Here's how the part is built. I have some questions about the finished solid (model axes, mm). Face numbers are marked on the shaded views. A direction names the side the tool comes from. Give positions to 0.01 mm unless a question says otherwise; leave off trailing zeros. Order: outer loops, then holes, each group sorted by start corner. A loop starts at its lowest first (then second) coordinate and runs counter-clockwise, first axis right, second up. Notation, with made-up numbers: (-5.5, -28.75) -> (34.5, -28.75) arc R36 ccw to (34.5, 7.25) -> close; hole circle Ø8 at (-13.5, 85.5). An arc over 180 degrees is marked (long way). Write each question's results on one line, items separated by ' | '. Start each with the question number.
Q1. Imagine slicing it at C-C, the plane x = -4.5. Please give me the cut outline in (y, z).
Q2. I need wall thicknesses on line 1 along X through (y, z) = (-10.5, 1.05); line 2 along Y through (x, z) = (15.25, -1.1); line 3 along Y through (x, z) = (15.25, 0.6). Which ranges of each line are inside material? Lowest first, please. Write a range as [from, to].
Q3. Imagine slicing it at B-B, the plane z = -3.15. State how many separate pieces and enclosed holes the cut face has, then the cut area to 3 significant figures.
Q4. Imagine slicing it at A-A, the plane y = -7.5. Please give me the cut outline in (x, z).
Q5. Thinking about a two-plate mould opening in X: for the marked faces 1, 2 and 3, which applies, pulls with the +X half, pulls with the -X half, needs draft (parallel to the pull), parting line crosses it, or undercut?
Q6. For the marked faces 4, 5 and 6, which set-ups out of +Z, -Z, +X, -X, +Y, -Y let a thin tool reach every point of the face, with its end or its side?
Q7. I'm going to push flat-ended pins straight in: pin 1 (2 mm diameter, centred on x = 4, z = -0.5, fed in from -Y); pin 2 (2 mm diameter, centred on y = 5, z = -2.5, fed in from -X); pin 3 (3 mm diameter, centred on x = 8, y = -2.5, fed in from -Z). Where does each tip first touch, or does it pass through?
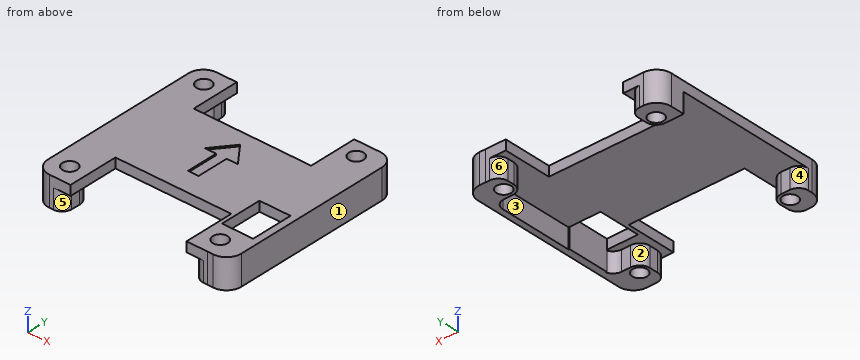
```python
from build123d import *

# Parameters (mm, degrees)
F0_R         = 1.5
F1_DEPTH     = 2
F2_DEPTH     = 4
F3_T1_DEPTH  = 9
F4_T4_DEPTH  = 9
F4_T6_DEPTH  = 4
F4_T8_DEPTH  = 9
F4_T10_DEPTH = 8.8612846748
F4_T12_DEPTH = 9
F4_T14_DEPTH = 9
F5_R         = 3
F6_R         = 3
F8_DEPTH     = 0.3


# Not quite as in the source:
# - a fillet or chamfer that OpenCascade refuses, or shapes differently, is made with other operations: its cross-section is extruded or revolved along the edge and cut away or added


with BuildPart() as f1:
    # F0 (on Top) → F1 (new body)
    with BuildSketch(Plane.XY):
        with BuildLine():
            Line((11.75, -19), (13.2, -19))
            Line((13.2, -19), (13.2, -15.25))
            ThreePointArc((13.2, -15.25), (13.8004310986, -13.8004310986), (15.25, -13.2))
            Line((15.25, -13.2), (19, -13.2))
            Line((19, -13.2), (19, -11.75))
            Line((19, -11.75), (18.8090763986, -11.75))
            Line((18.8090763986, -11.75), (12.5, -11.75))
            Line((12.5, -11.75), (12.5, -3.25))
            Line((12.5, -3.25), (18.8090763986, -3.25))
            Line((18.8090763986, -3.25), (19, -3.25))
            Line((19, -3.25), (19, 13.6544716179))
            Line((19, 13.6544716179), (15.25, 13.6544716179))
            ThreePointArc((15.25, 13.6544716179), (13.8004310986, 14.2549027165), (13.2, 15.7044716179))
            Line((13.2, 15.7044716179), (13.2, 19))
            Line((13.2, 19), (11.9, 19))
            Line((11.9, 19), (11.9, 9.2))
            Line((11.9, 9.2), (0, 9.2))
            Line((0, 9.2), (-11.9, 9.2))
            Line((-11.9, 9.2), (-11.9, 19))
            Line((-11.9, 19), (-13.2, 19))
            Line((-13.2, 19), (-13.2, 15.25))
            ThreePointArc((-13.2, 15.25), (-13.8004310986, 13.8004310986), (-15.25, 13.2))
            Line((-15.25, 13.2), (-19, 13.2))
            Line((-19, 13.2), (-19, -13.2))
            Line((-19, -13.2), (-15.25, -13.2))
            ThreePointArc((-15.25, -13.2), (-13.7801859172, -13.8209630649), (-13.2008111101, -15.3076618908))
            Line((-13.2008111101, -15.3076618908), (-13.304709388, -19))
            Line((-13.304709388, -19), (-11.75, -19))
            Line((-11.75, -19), (-11.75, -8.8))
            Line((-11.75, -8.8), (11.75, -8.8))
            Line((11.75, -8.8), (11.75, -19))
        make_face()
        with BuildLine():
            Line((-19, 16), (-19, 13.2))
            Line((-19, 13.2), (-15.25, 13.2))
            ThreePointArc((-15.25, 13.2), (-13.8004310986, 13.8004310986), (-13.2, 15.25))
            Line((-13.2, 15.25), (-13.2, 19))
            Line((-13.2, 19), (-16, 19))
            ThreePointArc((-16, 19), (-18.1213203436, 18.1213203436), (-19, 16))
        make_face()
        with Locations((-15.25, 15.25)):
            Circle(F0_R, mode=Mode.SUBTRACT)
        with BuildLine():
            Line((13.2, -19), (16, -19))
            Line((16, -19), (20.2087182552, -19.0532333363))
            Line((20.2087182552, -19.0532333363), (20.2087182552, 18.9976152033))
            Line((20.2087182552, 18.9976152033), (16, 19))
            Line((16, 19), (13.2, 19))
            Line((13.2, 19), (13.2, 15.7044716179))
            ThreePointArc((13.2, 15.7044716179), (13.8004310986, 14.2549027165), (15.25, 13.6544716179))
            Line((15.25, 13.6544716179), (19, 13.6544716179))
            Line((19, 13.6544716179), (19, -3.25))
            Line((19, -3.25), (18.8090763986, -3.25))
            Line((18.8090763986, -3.25), (18.8090763986, -11.75))
            Line((18.8090763986, -11.75), (19, -11.75))
            Line((19, -11.75), (19, -13.2))
            Line((19, -13.2), (15.25, -13.2))
            ThreePointArc((15.25, -13.2), (13.8004310986, -13.8004310986), (13.2, -15.25))
            Line((13.2, -15.25), (13.2, -19))
        make_face()
        with Locations((15.25, -15.25)):
            Circle(F0_R, mode=Mode.SUBTRACT)
        with Locations((15.25, 15.7044716179)):
            Circle(F0_R, mode=Mode.SUBTRACT)
        with BuildLine():
            Line((-16, -19), (-13.304709388, -19))
            Line((-13.304709388, -19), (-13.2008111101, -15.3076618908))
            ThreePointArc((-13.2008111101, -15.3076618908), (-13.7801859172, -13.8209630649), (-15.25, -13.2))
            Line((-15.25, -13.2), (-19, -13.2))
            Line((-19, -13.2), (-19, -16))
            ThreePointArc((-19, -16), (-18.1213203436, -18.1213203436), (-16, -19))
        make_face()
        with Locations((-15.25, -15.25)):
            Circle(F0_R, mode=Mode.SUBTRACT)
    extrude(amount=F1_DEPTH)

    # F0 (on Top) → F2 (join)
    with BuildSketch(Plane.XY):
        with BuildLine():
            Line((-16, -19), (-13.304709388, -19))
            Line((-13.304709388, -19), (-13.2008111101, -15.3076618908))
            ThreePointArc((-13.2008111101, -15.3076618908), (-13.7801859172, -13.8209630649), (-15.25, -13.2))
            Line((-15.25, -13.2), (-19, -13.2))
            Line((-19, -13.2), (-19, -16))
            ThreePointArc((-19, -16), (-18.1213203436, -18.1213203436), (-16, -19))
        make_face()
        with Locations((-15.25, -15.25)):
            Circle(F0_R, mode=Mode.SUBTRACT)
        with BuildLine():
            Line((13.2, -19), (16, -19))
            Line((16, -19), (20.2087182552, -19.0532333363))
            Line((20.2087182552, -19.0532333363), (20.2087182552, 18.9976152033))
            Line((20.2087182552, 18.9976152033), (16, 19))
            Line((16, 19), (13.2, 19))
            Line((13.2, 19), (13.2, 15.7044716179))
            ThreePointArc((13.2, 15.7044716179), (13.8004310986, 14.2549027165), (15.25, 13.6544716179))
            Line((15.25, 13.6544716179), (19, 13.6544716179))
            Line((19, 13.6544716179), (19, -3.25))
            Line((19, -3.25), (18.8090763986, -3.25))
            Line((18.8090763986, -3.25), (18.8090763986, -11.75))
            Line((18.8090763986, -11.75), (19, -11.75))
            Line((19, -11.75), (19, -13.2))
            Line((19, -13.2), (15.25, -13.2))
            ThreePointArc((15.25, -13.2), (13.8004310986, -13.8004310986), (13.2, -15.25))
            Line((13.2, -15.25), (13.2, -19))
        make_face()
        with Locations((15.25, -15.25)):
            Circle(F0_R, mode=Mode.SUBTRACT)
        with Locations((15.25, 15.7044716179)):
            Circle(F0_R, mode=Mode.SUBTRACT)
        with BuildLine():
            Line((-19, 16), (-19, 13.2))
            Line((-19, 13.2), (-15.25, 13.2))
            ThreePointArc((-15.25, 13.2), (-13.8004310986, 13.8004310986), (-13.2, 15.25))
            Line((-13.2, 15.25), (-13.2, 19))
            Line((-13.2, 19), (-16, 19))
            ThreePointArc((-16, 19), (-18.1213203436, 18.1213203436), (-19, 16))
        make_face()
        with Locations((-15.25, 15.25)):
            Circle(F0_R, mode=Mode.SUBTRACT)
    extrude(amount=-F2_DEPTH)

    # F3: fillet of radius 2 on 1 edges, made by hand

    # F3_s2 → F3_t1 (cut)
    with BuildSketch(Plane.XY.offset(-9)):
        with BuildLine():
            ThreePointArc((-13.2, 17), (-13.7857864376, 18.4142135624), (-15.2, 19))
            Line((-15.2, 19), (-13.2, 19))
            Line((-13.2, 19), (-13.2, 17))
        make_face()
    extrude(amount=F3_T1_DEPTH, mode=Mode.SUBTRACT)

    # F4: fillet of radius 2 on 6 edges, made by hand


with BuildPart() as f4_tool2:
    # F4_s3 → F4_t4 (new body)
    with BuildSketch(Plane.XY.offset(5)):
        with BuildLine():
            ThreePointArc((17, 13.6544716179), (18.4142135624, 13.0686851803), (19, 11.6544716179))
            Line((19, 11.6544716179), (19, 13.6544716179))
            Line((19, 13.6544716179), (17, 13.6544716179))
        make_face()
    extrude(amount=-F4_T4_DEPTH)

    split(bisect_by=Plane.XY.offset(2), keep=Keep.BOTTOM)


with BuildPart() as f1_1:
    add(f1.part)

    # F4_t1: union F4_tool2
    add(f4_tool2.part)

    # F4_s7 → F4_t6 (join)
    with BuildSketch(Plane.XY.offset(-4)):
        with BuildLine():
            ThreePointArc((17.0771115477, -13.2), (18.2812710056, -12.7968719423), (19, -11.75))
            Line((19, -11.75), (19, -13.2))
            Line((19, -13.2), (17.0771115477, -13.2))
        make_face()
    extrude(amount=F4_T6_DEPTH)

    # F4_s9 → F4_t8 (cut)
    with BuildSketch(Plane.XY.offset(-9)):
        with BuildLine():
            ThreePointArc((-19, -15.2), (-18.4142135624, -13.7857864376), (-17, -13.2))
            Line((-17, -13.2), (-19, -13.2))
            Line((-19, -13.2), (-19, -15.2))
        make_face()
    extrude(amount=F4_T8_DEPTH, mode=Mode.SUBTRACT)

    # F4_s11 → F4_t10 (cut)
    with BuildSketch(Plane.XY.offset(-8.8612846748)):
        with BuildLine():
            ThreePointArc((-13.2500145849, -17.0562555032), (-13.8550408822, -18.4339649588), (-15.249223258, -19))
            Line((-15.249223258, -19), (-13.304709388, -19))
            Line((-13.304709388, -19), (-13.2500145849, -17.0562555032))
        make_face()
    extrude(amount=F4_T10_DEPTH, mode=Mode.SUBTRACT)

    # F4_s13 → F4_t12 (cut)
    with BuildSketch(Plane.XY.offset(-9)):
        with BuildLine():
            ThreePointArc((13.2, 17), (13.7857864376, 18.4142135624), (15.2, 19))
            Line((15.2, 19), (13.2, 19))
            Line((13.2, 19), (13.2, 17))
        make_face()
    extrude(amount=F4_T12_DEPTH, mode=Mode.SUBTRACT)

    # F4_s15 → F4_t14 (cut)
    with BuildSketch(Plane.XY.offset(-9)):
        with BuildLine():
            ThreePointArc((13.2, -17), (13.7857864376, -18.4142135624), (15.2, -19))
            Line((15.2, -19), (13.2, -19))
            Line((13.2, -19), (13.2, -17))
        make_face()
    extrude(amount=F4_T14_DEPTH, mode=Mode.SUBTRACT)

    # F5
    f5_edges = [f1_1.edges().sort_by_distance(p)[0] for p in [
        (20.208718, -19.053233, -1),
    ]]
    fillet(f5_edges, radius=F5_R)

    # F6
    f6_edges = [f1_1.edges().sort_by_distance(p)[0] for p in [
        (20.208718, 18.997615, -1),
    ]]
    fillet(f6_edges, radius=F6_R)

    # F7 (on face) → F8 (cut)
    with BuildSketch(Plane.XY.offset(2)):
        Polygon((-1.0717540281, -4.259434063), (1.0717540281, -4.259434063), (1.0717540281, 2.1297170315), (3.3500560094, 2.1297170315), (0, 6.3891510945), (-3.3500560094, 2.1297170315), (-1.0717540281, 2.1297170315), align=None)
    extrude(amount=-F8_DEPTH, mode=Mode.SUBTRACT)


solid = f1_1.part
```
Geometry check:
1) outline: (-8.8, 0) -> (9.2, 0) -> (9.2, 2) -> (-8.8, 2) -> close
2) line 1: [-19, -11.75], [11.75, 12.5], [18.81, 20.21] | line 2: [-19, -16.75], [-13.75, -13.2], [13.65, 14.2], [17.2, 19] | line 3: [-19, -16.75], [-13.75, -11.75], [-3.25, 14.2], [17.2, 19]
3) separate pieces: 3 | enclosed holes: 4 | area: 137 mm²
4) outline: (-19, 0) -> (12.5, 0) -> (12.5, 2) -> (-19, 2) -> close; (18.81, -4) -> (20.21, -4) -> (20.21, 2) -> (18.81, 2) -> close
5) face 1: pulls with the +X half | face 2: undercut | face 3: pulls with the -X half
6) face 4: -Z, -X | face 5: -Z, -Y | face 6: -Z, +Y
7) pin 1: y = -8.8 | pin 2: x = 19 | pin 3: z = 0
